Model file for the job. Use its own axes, mm. A direction names the side the tool comes from. Give positions to 0.01 mm unless a question says otherwise; leave off trailing zeros. Write each loop counter-clockwise with the first axis right and the second up, starting at its lowest first coordinate (ties: lowest second). Pieces come first, ordered by that corner, then holes. Notation, with made-up numbers: (39, 14) - (80, 14) arc R24 cw to (80, 42) - close; hole circle Ø1 at (-24.5, 31.25). An arc over 180 degrees is marked (long way). Use CSV: the item, a comma, the result in double quotes.
from build123d import *

# Parameters (mm, degrees)
SKETCH_1_R          = 5
EXTRUDE_1_DEPTH     = 75
SKETCH_2_W          = 30
SKETCH_2_H          = 10
SKETCH_2_W_2        = 10
CUT_EXTRUDE_1_DEPTH = 0.5


with BuildPart() as part:
    # 草图1 → 凸台-拉伸1 (new body)
    with BuildSketch(Plane.XY):
        Circle(SKETCH_1_R)
    extrude(amount=EXTRUDE_1_DEPTH)

    # 草图2 → 切除-拉伸1 (cut)
    with BuildSketch(Plane(origin=(5, 0, 0), x_dir=(0, 0, -1), z_dir=(1, 0, 0))):
        with Locations((-37.5, 0)):
            Rectangle(SKETCH_2_W, SKETCH_2_H)
        with Locations((-70, 0)):
            Rectangle(SKETCH_2_W_2, SKETCH_2_H)
        with Locations((-5, 0)):
            Rectangle(SKETCH_2_W_2, SKETCH_2_H)
    extrude(amount=-CUT_EXTRUDE_1_DEPTH, mode=Mode.SUBTRACT)


solid = part.part
(1) Saw through at A-A, the plane y = 0. List the corners of the cut face in (x, z), then the cut area to 3 significant figures.
Checked values:
outline,"(-5, 0) - (4.5, 0) - (4.5, 10) - (5, 10) - (5, 22.5) - (4.5, 22.5) - (4.5, 52.5) - (5, 52.5) - (5, 65) - (4.5, 65) - (4.5, 75) - (-5, 75) - close"
area,"725 mm^2"
(2) Saw through at B-B, the plane z = 29.5. List the corners of the cut face in (x, y).
Checked values:
outline,"(4.5, -2.18) - (4.5, 2.18) arc R5 ccw (long way) to start"
(3) Wall check: probe 1 along X at (y, z) = (-2.75, 24.5); probe 2 along Y at (x, z) = (1.5, 54.5); probe 3 along X at (y, z) = (1, 33.5). Give the ranges that are in metal, low to high. Write a range as [from, to].
Checked values:
probe 1,"x = [-4.18, 4.18]"
probe 2,"y = [-4.77, 4.77]"
probe 3,"x = [-4.9, 4.5]"
(4) 3-axis set-ups, long thin cutter, end or side, ignore diameter. For faces 1 (the face through (-5, 0, 37)), 2 (the face through (4.5, 0, 70)): which of +Z, -Z, +X, -X, +Y, -Y reach the whole face in a straight line?
Checked values:
face 1,"+Z, -Z"
face 2,"+Z, +X, +Y, -Y"
(5) Flat gauge pins, fed straight in: P1, Ø1.5, axis at x = 4, z = 21, coming from the +Y side; P2, Ø2, axis at y = -0.5, z = 71.5, coming from the +X side. Where does each tip first touch, or does it go through?
Checked values:
P1,"stops at y = 3.8"
P2,"stops at x = 4.5"
(6) Saw through at D-D, the plane z = 59.5. List the corners of the cut face in (x, y), then the cut area to 3 significant figures.
Checked values:
outline,"circle Ø10 at (0, 0)"
area,"78.5 mm^2"
(7) Pull direction Z, two halves, no side cores. Call faces 3 (the face through (0, 0, 75)), 4 (the face through (0, 0, 0)), 5 (the face through (4.5, 0, 38)), 6 (the face through (4.5, 0, 5)): released by +Z, released by -Z, zero draft, split by the parting line, or undercut.
Checked values:
face 3,"released by +Z"
face 4,"released by -Z"
face 5,"undercut"
face 6,"zero draft"
(8) Saw through at C-C, the plane x = -1.75. List the corners of the cut face in (y, z), then the cut area to 3 significant figures.
Checked values:
outline,"(-4.68, 0) - (4.68, 0) - (4.68, 75) - (-4.68, 75) - close"
area,"703 mm^2"
